Geometry check sheet. Reference: the model listing, model coordinates, mm. A direction names the side the tool comes from. Coordinates: 2 decimals unless noted, no trailing zeros.
```python
from build123d import *

# Parameters (mm, degrees)
CYLINDER020_R           = 2
CYLINDER020_DEPTH       = 13
CYLINDER020_PITCH_ANGLE = 90
CYLINDER019_R           = 2
CYLINDER019_DEPTH       = 13
CYLINDER019_PITCH_ANGLE = 90
BOX002_W                = 19
BOX002_H                = 12
BOX002_DEPTH            = 25
CYLINDER017_R           = 2
CYLINDER017_DEPTH       = 25
CYLINDER018_R           = 2
CYLINDER018_DEPTH       = 25
CYLINDER015_R           = 1.5
CYLINDER015_DEPTH       = 25
CYLINDER016_R           = 3
CYLINDER016_DEPTH       = 25
CYLINDER013_R           = 1.5
CYLINDER013_DEPTH       = 25
CYLINDER014_R           = 3
CYLINDER014_DEPTH       = 25
CYLINDER012_R           = 1.75
CYLINDER012_DEPTH       = 25
CYLINDER011_R           = 1.75
CYLINDER011_DEPTH       = 25
CYLINDER010_R           = 1.75
CYLINDER010_DEPTH       = 25
CYLINDER002_R           = 2
CYLINDER002_DEPTH       = 25
CYLINDER003_R           = 2
CYLINDER003_DEPTH       = 25
CYLINDER004_R           = 2
CYLINDER004_DEPTH       = 25
CYLINDER005_R           = 2
CYLINDER005_DEPTH       = 25
CYLINDER006_R           = 3
CYLINDER006_DEPTH       = 25
CYLINDER007_R           = 3
CYLINDER007_DEPTH       = 25
CYLINDER008_R           = 5
CYLINDER008_DEPTH       = 25
CYLINDER009_R           = 5
CYLINDER009_DEPTH       = 25
BOX001_W                = 10
BOX001_H                = 10
BOX001_DEPTH            = 25
CYLINDER_R              = 2
CYLINDER_DEPTH          = 25
CYLINDER001_R           = 2
CYLINDER001_DEPTH       = 25
BOX_W                   = 300
BOX_H                   = 70
BOX_DEPTH               = 18


with BuildPart() as cilindro020:
    # Cylinder020 → Cylinder020 (new body)
    with BuildSketch(Plane.XY):
        Circle(CYLINDER020_R)
    extrude(amount=CYLINDER020_DEPTH)


with BuildPart() as cilindro020_1:
    # Cylinder020 pitch: moved
    add(cilindro020.part.rotate(Axis((0, 0, 0), (0, 1, 0)), CYLINDER020_PITCH_ANGLE))


with BuildPart() as cilindro020_2:
    # Cylinder020 placement: moved
    add(cilindro020_1.part.moved(Location((0, 60, 9))))


with BuildPart() as mirror_of_cilindro020:
    # mirror001: instance of Cilindro020
    add(cilindro020_2.part.mirror(Plane(origin=(300, 0, 18), x_dir=(0, -1, 0), z_dir=(1, 0, 0))))


with BuildPart() as mirror_of_cilindro020_1:
    # mirror001 placement: moved
    add(mirror_of_cilindro020.part.moved(Location((-300, 0, 0))))


with BuildPart() as cilindro019:
    # Cylinder019 → Cylinder019 (new body)
    with BuildSketch(Plane.XY):
        Circle(CYLINDER019_R)
    extrude(amount=CYLINDER019_DEPTH)


with BuildPart() as cilindro019_1:
    # Cylinder019 pitch: moved
    add(cilindro019.part.rotate(Axis((0, 0, 0), (0, 1, 0)), CYLINDER019_PITCH_ANGLE))


with BuildPart() as cilindro019_2:
    # Cylinder019 placement: moved
    add(cilindro019_1.part.moved(Location((0, 10, 9))))


with BuildPart() as mirror_of_cilindro019:
    # mirror: instance of Cilindro019
    add(cilindro019_2.part.mirror(Plane(origin=(300, 0, 18), x_dir=(0, -1, 0), z_dir=(1, 0, 0))))


with BuildPart() as mirror_of_cilindro019_1:
    # mirror placement: moved
    add(mirror_of_cilindro019.part.moved(Location((-300, 0, 0))))


with BuildPart() as cubo002:
    # Box002 → Box002 (new body)
    with BuildSketch(Plane(origin=(254.5, 48, 0), x_dir=(1, 0, 0), z_dir=(0, 0, 1))):
        with Locations((9.5, 6)):
            Rectangle(BOX002_W, BOX002_H)
    extrude(amount=BOX002_DEPTH)


with BuildPart() as cilindro017:
    # Cylinder017 → Cylinder017 (new body)
    with BuildSketch(Plane(origin=(288, 35, 0), x_dir=(1, 0, 0), z_dir=(0, 0, 1))):
        Circle(CYLINDER017_R)
    extrude(amount=CYLINDER017_DEPTH)


with BuildPart() as cilindro018:
    # Cylinder018 → Cylinder018 (new body)
    with BuildSketch(Plane(origin=(273.5, 35, 0), x_dir=(1, 0, 0), z_dir=(0, 0, 1))):
        Circle(CYLINDER018_R)
    extrude(amount=CYLINDER018_DEPTH)


with BuildPart() as cilindro015:
    # Cylinder015 → Cylinder015 (new body)
    with BuildSketch(Plane(origin=(150.5, 29, 0), x_dir=(1, 0, 0), z_dir=(0, 0, 1))):
        Circle(CYLINDER015_R)
    extrude(amount=CYLINDER015_DEPTH)


with BuildPart() as fusion002:
    # Cylinder016 → Cylinder016 (new body)
    with BuildSketch(Plane(origin=(150.5, 29, 11), x_dir=(1, 0, 0), z_dir=(0, 0, 1))):
        Circle(CYLINDER016_R)
    extrude(amount=CYLINDER016_DEPTH)

    # Fusion002: union Cilindro015
    add(cilindro015.part)


with BuildPart() as fusion002_1:
    # Fusion002 placement: moved
    add(fusion002.part.moved(Location((104, 0, 0))))


with BuildPart() as cilindro013:
    # Cylinder013 → Cylinder013 (new body)
    with BuildSketch(Plane(origin=(150.5, 29, 0), x_dir=(1, 0, 0), z_dir=(0, 0, 1))):
        Circle(CYLINDER013_R)
    extrude(amount=CYLINDER013_DEPTH)


with BuildPart() as fusion001:
    # Cylinder014 → Cylinder014 (new body)
    with BuildSketch(Plane(origin=(150.5, 29, 11), x_dir=(1, 0, 0), z_dir=(0, 0, 1))):
        Circle(CYLINDER014_R)
    extrude(amount=CYLINDER014_DEPTH)

    # Fusion001: union Cilindro013
    add(cilindro013.part)


with BuildPart() as cilindro012:
    # Cylinder012 → Cylinder012 (new body)
    with BuildSketch(Plane(origin=(137, 55, 0), x_dir=(1, 0, 0), z_dir=(0, 0, 1))):
        Circle(CYLINDER012_R)
    extrude(amount=CYLINDER012_DEPTH)


with BuildPart() as cilindro011:
    # Cylinder011 → Cylinder011 (new body)
    with BuildSketch(Plane(origin=(85, 50, 0), x_dir=(1, 0, 0), z_dir=(0, 0, 1))):
        Circle(CYLINDER011_R)
    extrude(amount=CYLINDER011_DEPTH)


with BuildPart() as cilindro010:
    # Cylinder010 → Cylinder010 (new body)
    with BuildSketch(Plane(origin=(85, 22, 0), x_dir=(1, 0, 0), z_dir=(0, 0, 1))):
        Circle(CYLINDER010_R)
    extrude(amount=CYLINDER010_DEPTH)


with BuildPart() as cilindro002:
    # Cylinder002 → Cylinder002 (new body)
    with BuildSketch(Plane(origin=(60, 20, 0), x_dir=(1, 0, 0), z_dir=(0, 0, 1))):
        Circle(CYLINDER002_R)
    extrude(amount=CYLINDER002_DEPTH)


with BuildPart() as cilindro003:
    # Cylinder003 → Cylinder003 (new body)
    with BuildSketch(Plane(origin=(60, 50, 0), x_dir=(1, 0, 0), z_dir=(0, 0, 1))):
        Circle(CYLINDER003_R)
    extrude(amount=CYLINDER003_DEPTH)


with BuildPart() as cilindro004:
    # Cylinder004 → Cylinder004 (new body)
    with BuildSketch(Plane(origin=(12, 35, 0), x_dir=(1, 0, 0), z_dir=(0, 0, 1))):
        Circle(CYLINDER004_R)
    extrude(amount=CYLINDER004_DEPTH)


with BuildPart() as cilindro005:
    # Cylinder005 → Cylinder005 (new body)
    with BuildSketch(Plane(origin=(26.5, 35, 0), x_dir=(1, 0, 0), z_dir=(0, 0, 1))):
        Circle(CYLINDER005_R)
    extrude(amount=CYLINDER005_DEPTH)


with BuildPart() as cilindro006:
    # Cylinder006 → Cylinder006 (new body)
    with BuildSketch(Plane(origin=(78, 15, 0), x_dir=(1, 0, 0), z_dir=(0, 0, 1))):
        Circle(CYLINDER006_R)
    extrude(amount=CYLINDER006_DEPTH)


with BuildPart() as cilindro007:
    # Cylinder007 → Cylinder007 (new body)
    with BuildSketch(Plane(origin=(78, 20, 0), x_dir=(1, 0, 0), z_dir=(0, 0, 1))):
        Circle(CYLINDER007_R)
    extrude(amount=CYLINDER007_DEPTH)


with BuildPart() as cilindro008:
    # Cylinder008 → Cylinder008 (new body)
    with BuildSketch(Plane(origin=(78, 35, 0), x_dir=(1, 0, 0), z_dir=(0, 0, 1))):
        Circle(CYLINDER008_R)
    extrude(amount=CYLINDER008_DEPTH)


with BuildPart() as cilindro009:
    # Cylinder009 → Cylinder009 (new body)
    with BuildSketch(Plane(origin=(78, 45, 0), x_dir=(1, 0, 0), z_dir=(0, 0, 1))):
        Circle(CYLINDER009_R)
    extrude(amount=CYLINDER009_DEPTH)


with BuildPart() as cubo001:
    # Box001 → Box001 (new body)
    with BuildSketch(Plane(origin=(73, 35, 0), x_dir=(1, 0, 0), z_dir=(0, 0, 1))):
        with Locations((5, 5)):
            Rectangle(BOX001_W, BOX001_H)
    extrude(amount=BOX001_DEPTH)


with BuildPart() as cilindro:
    # Cylinder → Cylinder (new body)
    with BuildSketch(Plane(origin=(10, 20, 0), x_dir=(1, 0, 0), z_dir=(0, 0, 1))):
        Circle(CYLINDER_R)
    extrude(amount=CYLINDER_DEPTH)


with BuildPart() as fusion:
    # Cylinder001 → Cylinder001 (new body)
    with BuildSketch(Plane(origin=(10, 50, 0), x_dir=(1, 0, 0), z_dir=(0, 0, 1))):
        Circle(CYLINDER001_R)
    extrude(amount=CYLINDER001_DEPTH)

    # Fusion: union Cilindro002, Cilindro003, Cilindro004, Cilindro005, Cilindro006, Cilindro007, Cilindro008, Cilindro009, Cubo001, Cilindro
    add(cilindro002.part)
    add(cilindro003.part)
    add(cilindro004.part)
    add(cilindro005.part)
    add(cilindro006.part)
    add(cilindro007.part)
    add(cilindro008.part)
    add(cilindro009.part)
    add(cubo001.part)
    add(cilindro.part)


with BuildPart() as cut012:
    # Box → Box (new body)
    with BuildSketch(Plane.XY):
        with Locations((150, 35)):
            Rectangle(BOX_W, BOX_H)
    extrude(amount=BOX_DEPTH)

    # Cut: cut Fusion
    add(fusion.part, mode=Mode.SUBTRACT)

    # Cut001: cut Cilindro010
    add(cilindro010.part, mode=Mode.SUBTRACT)

    # Cut002: cut Cilindro011
    add(cilindro011.part, mode=Mode.SUBTRACT)

    # Cut003: cut Cilindro012
    add(cilindro012.part, mode=Mode.SUBTRACT)

    # Cut004: cut Fusion001
    add(fusion001.part, mode=Mode.SUBTRACT)

    # Cut005: cut Fusion002
    add(fusion002_1.part, mode=Mode.SUBTRACT)

    # Cut006: cut Cilindro018
    add(cilindro018.part, mode=Mode.SUBTRACT)

    # Cut007: cut Cilindro017
    add(cilindro017.part, mode=Mode.SUBTRACT)

    # Cut008: cut Cubo002
    add(cubo002.part, mode=Mode.SUBTRACT)

    # Cut009: cut Cilindro019
    add(cilindro019_2.part, mode=Mode.SUBTRACT)

    # Cut010: cut Cilindro020
    add(cilindro020_2.part, mode=Mode.SUBTRACT)

    # Cut011: cut Mirror of Cilindro019
    add(mirror_of_cilindro019_1.part, mode=Mode.SUBTRACT)

    # Cut012: cut Mirror of Cilindro020
    add(mirror_of_cilindro020_1.part, mode=Mode.SUBTRACT)


solid = cut012.part
```
Item 1: Depth check by flat-ended pin: P1, Ø3, axis at x = 253.5, y = 30, coming from the +Z side; P2, Ø3, axis at y = 59.5, z = 9.5, coming from the -X side; P3, Ø3.5, axis at y = 10, z = 9, coming from the +X side. Enter the tip coordinate at first touch or a pass-through.
Item 2: Sectioned sample at A-A (z = 13.5). Give the number of separate pieces and of enclosed holes in the cut face, and give its area (3 significant figures).
Item 3: Release check for a two-part mould opening along X. For faces 1 (the face through (148, 0, 9)), 2 (the face through (300, 35, 9)), 3 (the face through (78, 30, 9)) record: pulls with the +X half, pulls with the -X half, needs draft (parallel to the pull), parting line crosses it, or undercut.
Item 4: Thickness scan on line 1 along X through (y, z) = (29, 3.75); line 2 along Y through (x, z) = (85, 5.25); line 3 along Y through (x, z) = (137, 8.25). Record the ranges inside material, lowest first.
Item 5: Tool access check on faces 4 (the face through (251.5, 29.1, 14.5)), 5 (the face through (148, 70, 9)), 6 (the face through (83, 40, 9)). Record the directions out of +Z, -Z, +X, -X, +Y, -Y that give a thin tool (end or side, any length) a straight path to the whole face; none if there is none.
Geometry check:
1. P1: stops at z = 11
1. P2: stops at x = 0
1. P3: stops at x = 287
2. separate pieces: 1
2. enclosed holes: 16
2. area: 20,400 mm2
3. face 1: needs draft
3. face 2: pulls with the +X half
3. face 3: undercut
4. line 1: x = 0 to 149, 152 to 253, 256 to 300
4. line 2: y = 0 to 20.25, 23.75 to 48.25, 51.75 to 70
4. line 3: y = 0 to 53.25, 56.75 to 70
5. face 4: +Z
5. face 5: +Z, -Z, +X, -X, +Y
5. face 6: +Z, -Z
